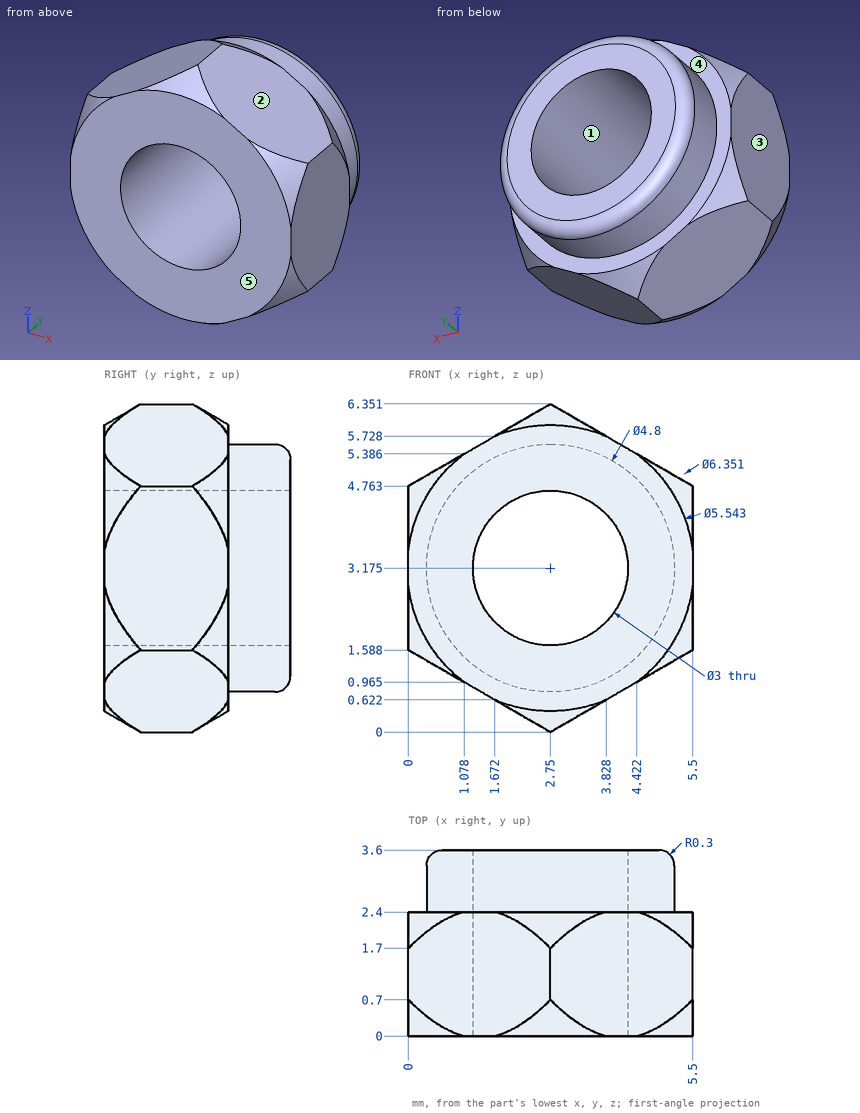
Answer from the drawing. Dimensions are ordinates in mm from the lowest x, y and z of the part. A direction names the side the tool comes from. Give positions to 0.01 mm unless a question says otherwise; leave off trailing zeros.
Item 1: A tool of negligible diameter and unlimited length cuts with its end or side. For the marked faces 4 and 5, from which of +Z, -Z, +X, -X, +Y, -Y can it reach the whole face along a straight path? Write none if from no direction.
Derived:
face 4: +Y
face 5: +Z, -Z, +X, -X, -Y
Item 2: Find the intervals of material crossed by line 1 along Y through (x, z) = (1.9, 5.75); line 2 along X through (y, z) = (0.4, 4) (1 decimal); line 3 along Z through (x, y) = (1.45, 3.15) (1 decimal), in increasing order.
Derived:
line 1: y = 0 to 2.4
line 2: x = 0 to 1.5, 4 to 5.5
line 3: z = 1.2 to 2.4, 3.9 to 5.2
Item 3: Determine the mould class of the marked faces 1, 2 and 3 for opening direction X: +X half, -X half, draft (parallel to the pull), parting line (faces both ways), or undercut.
Derived:
face 1: undercut
face 2: +X half
face 3: -X half
